Autodesk Inventor part; units mm, degrees
ref_plane "Work Plane1" through (-22.2692, 0, 0) normal (0, -0.866, -0.5) x (1, 0, 0)
ref_plane "YZ Plane" through (0, 0, 0) normal (1, 0, 0) x (0, 1, 0)
ref_plane "XZ Plane" through (0, 0, 0) normal (0, 1, 0) x (-1, 0, 0)
sketch "Sketch1" plane through (0, 0, 0) normal (1, 0, 0) x (0, 1, 0)
  line L0 (-12.1244, 0) -> (-6.0622, 10.5)
  line L1 (-6.0622, 10.5) -> (6.0622, 10.5)
  line L2 (6.0622, 10.5) -> (12.1244, 0)
  line L3 (12.1244, 0) -> (6.0622, -10.5)
  line L4 (6.0622, -10.5) -> (-6.0622, -10.5)
  line L5 (-6.0622, -10.5) -> (-12.1244, 0)
  point P0 (0, 0)
  point P1 (0, 0)
  dimension "d0" = 24.2487
extrude "Body" add sketch "Sketch1" along normal blind 12.3
sketch "Sketch2" plane through (0, 0, 0) normal (0, 0, 1) x (1, 0, 0)
  line L0 (0, 6.0622) -> (0, 12.1244)
  line L1 (0, 12.1244) -> (12.3, 12.1244)
  line L2 (12.3, 6.0622) -> (12.3, 12.1244)
  line L3 (-2.46, 0) -> (14.76, 0)
  line L4 (1.4574, 12.1244) -> (0, 9.6)
  line L5 (10.8426, 12.1244) -> (12.3, 9.6)
  dimension "d3" = 30
  dimension "d4" = 30
  dimension "d5" = 19.2
  dimension "d6" = 19.2
revolve "Chamfer1" cut sketch "Sketch2" angle 360 about axis through (-10, 0, 0) along (1, 0, 0)
sketch "Sketch3" plane through (12.3, 0, 0) normal (1, 0, 0) x (0, 0, -1)
  arc A0 (-0.625, -1.0825) -> (0.625, -1.0825) centre (0, 0) ccw
hole "Thread" at (12.3, 0, 0) direction (-1, 0, 0) diameter 10.106 end through all
chamfer "Chamfer2" distance 0.9472 angle 30 1 edges at (12.3, 0, 5.053) measured on face at (12.3, 7.9791, -0.9688)
chamfer "Chamfer3" distance 0.9472 angle 30 1 edges at (0, 0, 5.053) measured on face at (0, 7.9791, -0.9688)
ref_plane "Work Plane1" through (-22.2692, 0, 0) normal (0, -0.866, -0.5) x (1, 0, 0)
equation "\"d0\" = 1.1547 * SW"
equation "\"d1\" = KOH"
equation "\"d8\" = -0.5 * GD1 + 0.5 * NND"
equation "\"d40\" = -0.5 * GD1 + 0.5 * NND"
equation "\"d10\" = -0.5 * GD1 + 0.5 * NND"
equation "\"d41\" = -0.5 * GD1 + 0.5 * NND"
equation "\"d3\" = ANG1"
equation "\"d4\" = ANG2"
equation "\"d5\" = SW0"
equation "\"d6\" = SW01"
equation "\"ANG1\" = 30deg"
equation "\"ANG2\" = 30deg"
equation "\"NND\" = 12"
equation "\"KOH\" = 12.3"
equation "\"SW\" = 21"
equation "\"SW0\" = 19.2"
equation "\"SW01\" = SW0"
equation "\"GUL\" = 0.541266 * PTC"
equation "\"THREADDIA\" = 12"
equation "\"TOA\" = 30deg"
equation "\"PTC\" = 1.75"
equation "\"E0\" = 1.155 * SW"
equation "\"GAL\" = 0.541266 * PTC"
properties part number "ISO 4775 - M12" material "Steel"
Read the model definition and answer for the solid it produces. Units are mm, in the model's axes. Coordinates: 2 decimals unless noted, no trailing zeros. Write each loop counter-clockwise with the first axis right and the second up, starting at its lowest first coordinate (ties: lowest second). Pieces come first, ordered by that corner, then holes. Notation, with made-up numbers: (46, -10) -> (75, -10) arc R17 ccw to (75, 0) -> close; hole circle Ø5 at (57, 30.25). An arc over 180 degrees is marked (long way). Return JSON: item names as keys, results as strings.
(1) The part is cut by section A-A on x = 7.5. Give the vertices of the cut face in (y, z).
Answers below:
{"outline": "(-12.12, 0) -> (-6.06, -10.5) -> (6.06, -10.5) -> (12.12, 0) -> (6.06, 10.5) -> (-6.06, 10.5) -> close; hole circle Ø10.11 at (0, 0)"}
(2) For a pull along Z with two mould halves and no side action, classify faces 1 (the cylindrical face through (6.072, 3.075, 4.01)), 2 (the flat face through (6, 0, -10.5)), 3 (the flat face through (0, -0.1, -6.3)) as pulls with the +Z half, pulls with the -Z half, needs draft (parallel to the pull), parting line crosses it, or undercut.
Answers below:
{"face 1": "undercut", "face 2": "pulls with the -Z half", "face 3": "needs draft"}
(3) Consider line 1 along Z through (x, y) = (3, 0); line 2 along Z through (x, y) = (10.5, 3); line 3 along Y through (x, z) = (7, -3). Determine where each line is inside the solid, lowest interval first. Write a range as from..to.
Answers below:
{"line 1": "-10.5..-5.05, 5.05..10.5", "line 2": "-10.5..-4.07, 4.07..10.5", "line 3": "-10.39..-4.07, 4.07..10.39"}
(4) The part is cut by section B-B on y = 0. Give the vertices of the cut face in (x, z), then the cut area to 3 significant figures.
Answers below:
{"outline": "(0, -9.6) -> (0.52, -10.5) -> (11.78, -10.5) -> (12.3, -9.6) -> (12.3, -6) -> (11.75, -5.05) -> (0.55, -5.05) -> (0, -6) -> close; (0, 6) -> (0.55, 5.05) -> (11.75, 5.05) -> (12.3, 6) -> (12.3, 9.6) -> (11.78, 10.5) -> (0.52, 10.5) -> (0, 9.6) -> close", "area": "132 mm^2"}
(5) Each of these flat-tipped pins is pushed along its axis until it touches: P1, Ø2, axis at x = 9.5, z = 6.5, coming from the +Y side; P2, Ø8, axis at y = 0, z = 0, coming from the +X side. Where does it stop, or does it pass through?
Answers below:
{"P1": "y = 8.95", "P2": "through"}
